Autodesk Fusion 360 part; units mm, degrees
sketch "Sketch2" plane through (0, 0, 0) normal (0, 1, 0) x (1, 0, 0)
  line L0 (-80, 30) -> (-40, 30)
  line L1 (-40, 30) -> (4.2788, 9.0384)
  arc A0 (4.2788, -9.0384) -> (4.2788, 9.0384) centre (0, 0) ccw
  line L2 (4.2788, -9.0384) -> (-40, -30)
  line L3 (-40, -30) -> (-80, -30)
  circle A1 centre (0, 0) radius 6
  line L4 (-80, -10) -> (-60, -10)
  arc A2 (-60, -10) -> (-60, 10) centre (-60, 0) ccw
  line L5 (-60, 10) -> (-80, 10)
  line L6 (-80, -30) -> (-80, -10)
  line L7 (-80, 10) -> (-80, 30)
  line L8 (0, 0) -> (-89, 0) construction
  dimension "d22" = 12
  dimension "d23" = 10
  dimension "d24" = 20
  dimension "d25" = 20
  dimension "d26" = 40
  dimension "d27" = 60
  dimension "d28" = 80
  dimension "d29" = 10
extrude "Extrude2" add sketch "Sketch2" along normal blind 20
Source: CAD feature listing. Evaluate the final solid. Frame: model axes, mm. A direction names the side the tool comes from. Round coordinates to 2 decimals unless told otherwise and drop trailing zeros. Loops run counter-clockwise (first coordinate to the right, second up) from the corner with the lowest first, then second, coordinate; pieces in that order, holes last.
Q1. Section B-B, the plane x = -65. Return loops of the section in (y, z), plus the area to 3 significant figures.
Q2. Access query for faces 1 (the face through (-46, 0, 0)), 2 (the face through (-70, 10, -10)). Directions: +Z, -Z, +X, -X, +Y, -Y. A direction counts if a zero-diameter tool reaches every point of the face in a straight line with its end or side. Return the directions, or none.
Q3. First-contact query: P1, Ø8, axis at y = 8.5, z = -2.5, coming from the +X side; P2, Ø8, axis at x = -35, y = 8.5, coming from the +Z side; P3, Ø1.5, axis at y = 11.5, z = -8, coming from the +X side. Flat tips, straight axial feed; report the tip coordinate or a pass-through.
Q4. Section D-D, the plane z = -19. Return loops of the section in (x, y).
Q5. Section C-C, the plane z = 0. Return loops of the section in (x, y), plus the area to 3 significant figures.
Q6. Section A-A, the plane y = 12. Return loops of the section in (x, z).
Q7. Ray query, line 1 (Z direction, x = -61, y = 6.5); line 2 (Z direction, x = -1, y = 11.5); line 3 (X direction, y = 9, z = -22). Return the intervals inside material, ascending.
Solutions:
1. outline: (0, -30) - (20, -30) - (20, -10) - (0, -10) - close; (0, 10) - (20, 10) - (20, 30) - (0, 30) - close
1. area: 800 mm2
2. face 1: +Z, -Z, +X, -X, -Y
2. face 2: -X, +Y, -Y
3. P1: stops at x = 10
3. P2: stops at z = 29.53
3. P3: stops at x = 6.89
4. outline: (-80, 0) - (-16.76, 0) - (-16.76, 20) - (-80, 20) - close
5. outline: (-50, 0) - (-6, 0) - (-6, 20) - (-50, 20) - close; (6, 0) - (10, 0) - (10, 20) - (6, 20) - close
5. area: 960 mm2
6. outline: (-80, -30) - (-40, -30) - (4.28, -9.04) arc R10 ccw to (4.28, 9.04) - (-40, 30) - (-80, 30) - (-80, 10) - (-60, 10) arc R10 cw to (-60, -10) - (-80, -10) - close; hole circle Ø12 at (0, 0)
7. line 1: z = -30 to -10, 10 to 30
7. line 2: z = -11.54 to -5.92, 5.92 to 11.54
7. line 3: x = -80 to -23.1
